CAD build for the part. Positions are in the model's coordinates, mm. A direction names the side the tool comes from. Coordinates: 2 decimals unless noted, no trailing zeros. Loops run counter-clockwise (first coordinate to the right, second up) from the corner with the lowest first, then second, coordinate; pieces in that order, holes last. Notation, with made-up numbers: (-9, 84) -> (3, 84) arc R23 cw to (3, 99) -> close; hole circle Ø7 at (15, 34.5). An arc over 180 degrees is marked (long way). Write item = value, one per line. Start each with the question number.
(1) Band-saw the part on A-A (x = -27). Write the cut outline in (y, z), and give its area (3 significant figures).
(2) Tool access for faces 4 (the face through (9.088, 10, 1)), 5 (the face through (-25.74, 12.3, 1.01)), 6 (the face through (-46, 28.372, 1)): list every direction of +Z, -Z, +X, -X, +Y, -Y with a clear straight run to the whole face (end or side of a thin tool).
(3) Drill centre lines: line 1 (Y direction, x = -4, z = 1.65); line 2 (Y direction, x = -9, z = 1.65); line 3 (Y direction, x = -38.5, z = 1.3). Where is each one in solid material? Low to high. Write a range as from..to.
(4) Flat gauge pins, fed straight in: P1, Ø1, axis at y = 9, z = 0.5, coming from the +X side; P2, Ø0.6, axis at y = 26, z = 1.5, coming from the -X side. Where does each tip first touch, or does it go through?
(5) Band-saw the part on B-B (z = 1.4). Count the separate pieces of the cut face and the enclosed holes in it, and give its area (3 significant figures).
(6) Band-saw the part on C-C (y = -7). Write the cut outline in (x, z), and give its area (3 significant figures).
(7) Pull direction Y, two halves, no side cores. Call faces 1 (the face through (-18, -11.028, 1)), 2 (the face through (-10.4, 12.1, 1)), 3 (the face through (-46.912, 19.5, 1)): +Y half, -Y half, draft (parallel to the pull), parting line (faces both ways), or undercut.
```python
from build123d import *

# Parameters (mm, degrees)
SKETCH1_W               = 54
SKETCH1_H               = 37.4
BOSS_EXTRUDE1_DEPTH     = 2
CUT_EXTRUDE1_DEPTH      = 54.160020758
BOSS_EXTRUDE2_DEPTH     = 2
SKETCH4_W               = 2
SKETCH4_H               = 2
BOSS_EXTRUDE3_DEPTH     = 2
FILLET3_R               = 0.8
MIRROR5_COPY_1_SKETCH_W = 2
MIRROR5_COPY_1_SKETCH_H = 2
MIRROR5_COPY_1_DEPTH    = 2
FILLET3_OF_MIRROR5_R    = 0.8


with BuildPart() as part:
    # Sketch1 → Boss-Extrude1 (new body)
    with BuildSketch(Plane.XY):
        with Locations((-17.911518112, 9.671523538)):
            Rectangle(SKETCH1_W, SKETCH1_H)
    extrude(amount=BOSS_EXTRUDE1_DEPTH)

    # Sketch2 → Cut-Extrude1 (cut, through all)
    with BuildSketch(Plane.XY.offset(2)):
        Polygon((-22.764922959, 24.371523538), (-29.981326879, 19.759300163), (-37.197730799, 24.371523538), align=None)
        Polygon((-33.695114192, 17.385705663), (-40.911518112, 12.773482289), (-40.911518112, 21.997929038), align=None)
        Polygon((-29.981326879, 15.012111163), (-37.408901505, 10.264922163), (-29.052880051, 4.924334538), (-21.625305425, 9.671523538), align=None)
        Polygon((-18.83996494, 22.132894663), (-26.267539566, 17.385705663), (-17.911518112, 12.045118038), (-10.483943486, 16.792307038), align=None)
        Polygon((1.374694575, 24.371523538), (-14.915006921, 24.371523538), (-6.770156173, 19.165901538), align=None)
        Polygon((-3.05636886, 16.792307038), (5.088481888, 11.586685039), (5.088481888, 21.997929038), align=None)
        Polygon((-6.770156173, 14.418712538), (-14.197730799, 9.671523538), (-5.841709344, 4.330935913), (1.585865282, 9.078124913), align=None)
        Polygon((-17.911518112, 7.297929038), (-25.339092738, 2.550740038), (-16.983071283, -2.789847587), (-9.555496657, 1.957341413), align=None)
        Polygon((-29.052880051, 0.177145538), (-20.908029303, -5.028476462), (-37.197730799, -5.028476462), align=None)
        Polygon((-40.911518112, 7.756362038), (-32.766667364, 2.550740038), (-40.911518112, -2.654881962), align=None)
        Polygon((-13.058113264, -5.028476462), (-5.841709344, -0.416253087), (1.374694575, -5.028476462), align=None)
        Polygon((-2.127922031, 1.957341413), (5.088481888, 6.569564788), (5.088481888, -2.654881962), align=None)
    extrude(amount=-CUT_EXTRUDE1_DEPTH, mode=Mode.SUBTRACT)

    # Sketch3 → Boss-Extrude2 (add)
    with BuildSketch(Plane.XZ.offset(9.028476462)):
        Polygon((9.088481888, 2), (11.088481888, 2), (11.088481888, 0), (9.088481888, 0), (-44.911518112, 0), (-46.911518112, 0), (-46.911518112, 2), (-44.911518112, 2), align=None)
    boss_extrude2 = extrude(amount=BOSS_EXTRUDE2_DEPTH)

    # Sketch4 → Boss-Extrude3 (add)
    with BuildSketch(Plane(origin=(9.088481888, 0, 0), x_dir=(0, 0, -1), z_dir=(1, 0, 0))):
        with Locations((-1, 0.271523538)):
            Rectangle(SKETCH4_W, SKETCH4_H)
    boss_extrude3 = extrude(amount=BOSS_EXTRUDE3_DEPTH)

    # Mirror2: Boss-Extrude3 across plane
    add(boss_extrude3.mirror(Plane.ZY.offset(17.911518112)))

    # Fillet3
    fillet3_edges = [part.edges().sort_by_distance(p)[0] for p in [
        (9.088481888, 1.271523538, 1),
        (11.088481888, 1.271523538, 1),
        (-46.911518112, 1.271523538, 1),
        (-44.911518112, 1.271523538, 1),
        (-46.911518112, -11.028476462, 1),
        (11.088481888, -11.028476462, 1),
    ]]
    fillet(fillet3_edges, radius=FILLET3_R)

    # Mirror5: Boss-Extrude2, Boss-Extrude3 across plane
    add(boss_extrude2.mirror(Plane(origin=(0, 9.671523538, 0), x_dir=(0, 0, 1), z_dir=(0, -1, 0))))
    add(boss_extrude3.mirror(Plane(origin=(0, 9.671523538, 0), x_dir=(0, 0, 1), z_dir=(0, -1, 0))))

    # Mirror5 copy 1 sketch → Mirror5 copy 1 (add)
    with BuildSketch(Plane(origin=(-44.911518112, 19.343047076, 0), x_dir=(0, 0, -1), z_dir=(-1, 0, 0))):
        with Locations((-1, 0.271523538)):
            Rectangle(MIRROR5_COPY_1_SKETCH_W, MIRROR5_COPY_1_SKETCH_H)
    extrude(amount=MIRROR5_COPY_1_DEPTH)

    # Fillet3 of Mirror5
    fillet3_of_mirror5_edges = [part.edges().sort_by_distance(p)[0] for p in [
        (9.088481888, 18.071523538, 1),
        (11.088481888, 18.071523538, 1),
        (-46.911518112, 18.071523538, 1),
        (-44.911518112, 18.071523538, 1),
        (-46.911518112, 30.371523538, 1),
        (11.088481888, 30.371523538, 1),
    ]]
    fillet(fillet3_of_mirror5_edges, radius=FILLET3_OF_MIRROR5_R)


solid = part.part
```
Findings below:
q1.outline = (-11.03, 0) -> (-5.03, 0) -> (-5.03, 2) -> (-11.03, 2) -> close; (-1.13, 0) -> (6.24, 0) -> (6.24, 2) -> (-1.13, 2) -> close; (13.11, 0) -> (21.66, 0) -> (21.66, 2) -> (13.11, 2) -> close; (24.37, 0) -> (30.37, 0) -> (30.37, 2) -> (24.37, 2) -> close
q1.area = 55.9 mm²
q2.face_4 = +Z, -Z, +X
q2.face_5 = +Z, -Z
q2.face_6 = +Z, -Z, -X
q3.line_1 = -11.03..-5.03, -1.59..5.51, 12.65..20.94, 24.37..30.37
q3.line_2 = -11.03..-5.03, -2.43..6.35, 12.99..20.59, 24.37..30.37
q3.line_3 = -11.03..-1.11, 6.22..14.31, 20.46..30.37
q4.P1 = 9.09
q4.P2 = -44.91
q5.separate_pieces = 1
q5.enclosed_holes = 12
q5.area = 1,650 mm²
q6.outline = (-44.91, 0) -> (9.09, 0) -> (9.09, 2) -> (-44.91, 2) -> close
q6.area = 108 mm²
q7.face_1 = -Y half
q7.face_2 = undercut
q7.face_3 = draft
